Study the drawing (mm; zero at the part's minimum x, y, z) and answer. A direction names the side the tool comes from. Coordinates: 2 decimals unless noted, no trailing zeros. Order: outer loops, then holes, each group sorted by start corner. A loop starts at its lowest first (then second) coordinate and runs counter-clockwise, first axis right, second up.
1. The part is cut by section B-B, the plane y = 4. Give the vertices of the cut face in (x, z), then the cut area to 3 significant figures.
2. The part is cut by section C-C, the plane x = 8.5. Give the vertices of the cut face in (y, z), then the cut area to 3 significant figures.
3. The part is cut by section A-A, the plane z = 13. Give the vertices of the cut face in (x, y), then the cut area to 3 significant figures.
4. A tool of negligible diameter and unlimited length cuts with its end or side. For the marked faces 4 and 5, from which of +Z, -Z, +X, -X, +Y, -Y can it reach the whole face along a straight path? Write none if from no direction.
5. A flat-ended cylindrical pin translates along its axis: pin 1 Ø6 at (x, z) = (11, 12.5) entering from -Y. Find the tip coordinate at first contact, or state that the pin passes through.
6. The part is cut by section D-D, the plane z = 10.75. Give the vertices of the cut face in (x, y), then the cut area to 3 significant figures.
7. Find the intervals of material crossed by probe 1 along Z at (x, y) = (4, 7); probe 2 along X at (y, z) = (4.25, 4.5); probe 3 along Z at (x, y) = (8, 6.5), in increasing order.
8. Determine the mould class of the marked faces 1, 2 and 3 for opening direction Z: +Z half, -Z half, draft (parallel to the pull), parting line (faces both ways), or undercut.
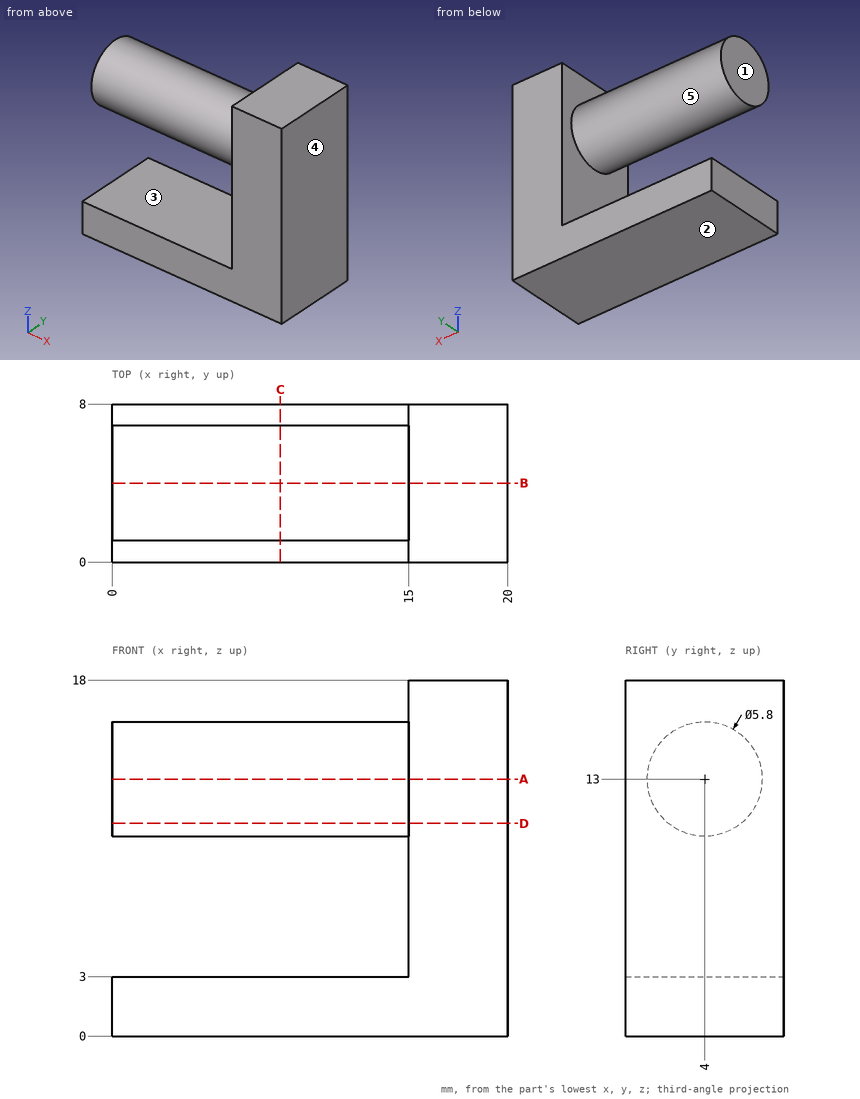
Geometry says:
1. outline: (0, 0) - (20, 0) - (20, 18) - (15, 18) - (15, 15.9) - (0, 15.9) - (0, 10.1) - (15, 10.1) - (15, 3) - (0, 3) - close
1. area: 222 mm2
2. outline: (0, 0) - (8, 0) - (8, 3) - (0, 3) - close; circle Ø5.8 at (4, 13)
2. area: 50.4 mm2
3. outline: (0, 1.1) - (15, 1.1) - (15, 0) - (20, 0) - (20, 8) - (15, 8) - (15, 6.9) - (0, 6.9) - close
3. area: 127 mm2
4. face 4: +Z, -Z, +X, +Y, -Y
4. face 5: -X
5. pin 1: stops at y = 1.1
6. outline: (0, 2.17) - (15, 2.17) - (15, 0) - (20, 0) - (20, 8) - (15, 8) - (15, 5.83) - (0, 5.83) - close
6. area: 94.9 mm2
7. probe 1: z = 0 to 3
7. probe 2: x = 15 to 20
7. probe 3: z = 0 to 3, 11.53 to 14.47
8. face 1: draft
8. face 2: -Z half
8. face 3: undercut
